Could you check a few things on this model? Use its own coordinates, in mm. Face numbers are marked on the shaded views. Round coordinates to 2 decimals unless told otherwise and drop trailing zeros. Loops run counter-clockwise (first coordinate to the right, second up) from the corner with the lowest first, then second, coordinate; pieces in that order, holes last. Notation, with made-up numbers: (-4, 21) -> (22, 21) arc R31 ccw to (22, 56) -> close; hole circle Ø10 at (76, -25). An arc over 180 degrees is marked (long way). Write each question's results on one line, items separated by ' | '. Start each with the question number.
1) Imagine slicing it at C-C, the plane y = 2.25. List the corners of the cut face in (x, z) for me.
2) We'd pull the mould along Y, two halves only. Please class the marked faces 1, 2 and 3: pulls with the +Y half, pulls with the -Y half, needs draft (parallel to the pull), parting line crosses it, or undercut.
3) If I drill on probe 1 along X at (y, z) = (-0.2, 3.17); probe 2 along X at (y, z) = (0.45, -1.91); probe 3 along Z at (x, y) = (4.5, -0.15), over which ranges is the centre line in solid material (lowest first)?
4) Imagine slicing it at D-D, the plane z = 0.63. Give the number of separate pieces and of enclosed holes in the cut face, plus the area to 3 significant figures.
5) Imagine slicing it at B-B, the plane x = 3.25. List the corners of the cut face in (y, z) for me.
6) Imagine slicing it at A-A, the plane z = -4.45. List the corners of the cut face in (x, y) for me, plus the area to 3 significant figures.
7) For P1, Ø1.5, axis at x = 0, z = -8, coming from the -Y side; P2, Ø1.8, axis at x = 7.5, z = 0.5, coming from the +Y side; P3, Ø2, axis at x = -6, y = 0.5, coming from the -Z side, each with a flat end and sliding along its axis, tell me the tip position at first contact or that it passes through.
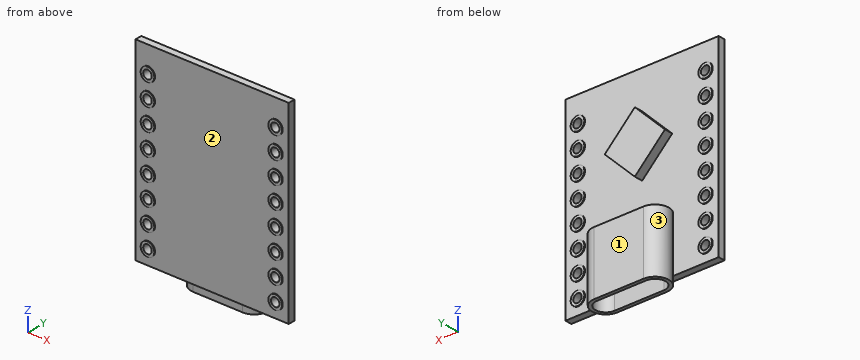
from build123d import *

# Parameters (mm, degrees)
SKETCH1_W                = 18
SKETCH1_H                = 22.5
BOSS_EXTRUDE1_DEPTH      = 0.4
CUT_EXTRUDE1_DEPTH       = 15.429223818
CUT_EXTRUDE1_DEPTH_BACK  = 15.429223818
SKETCH2_R                = 0.5
BOSS_EXTRUDE2_DEPTH      = 1.35
BOSS_EXTRUDE2_DEPTH_BACK = 6
CUT_EXTRUDE2_DEPTH       = 26.744562533
CUT_EXTRUDE2_DEPTH_BACK  = 7
BOSS_EXTRUDE3_DEPTH      = 1
BOSS_EXTRUDE4_DEPTH      = 0.1
BOSS_EXTRUDE4_DEPTH_BACK = 0.9
SKETCH6_R                = 0.8
SKETCH6_R_2              = 0.5


with BuildPart() as part:
    # Sketch1 → Boss-Extrude1 (new, symmetric)
    with BuildSketch(Plane(origin=(0, 0, 0), x_dir=(1, 0, 0), z_dir=(0, 1, 0))):
        Rectangle(SKETCH1_W, SKETCH1_H)
    extrude(amount=BOSS_EXTRUDE1_DEPTH, both=True)

    # Sketch2 → Cut-Extrude1 (cut, two sides: drawn at the far end of the back side and taken through both)
    with BuildSketch(Plane(origin=(0, 0.4, 0), x_dir=(1, 0, 0), z_dir=(0, 1, 0)).offset(-CUT_EXTRUDE1_DEPTH_BACK)):
        with Locations(Location((7.5, -8.25, 0), (0, 0, 270))):
            Circle(SKETCH2_R)
        with Locations(Location((-7.5, -8.25, 0), (0, 0, 270))):
            Circle(SKETCH2_R)
        with Locations(Location((-7.5, -5.71, 0), (0, 0, 270))):
            Circle(SKETCH2_R)
        with Locations(Location((7.5, -5.71, 0), (0, 0, 270))):
            Circle(SKETCH2_R)
        with Locations(Location((-7.5, -3.17, 0), (0, 0, 270))):
            Circle(SKETCH2_R)
        with Locations(Location((7.5, -3.17, 0), (0, 0, 270))):
            Circle(SKETCH2_R)
        with Locations(Location((-7.5, -0.63, 0), (0, 0, 270))):
            Circle(SKETCH2_R)
        with Locations(Location((7.5, -0.63, 0), (0, 0, 270))):
            Circle(SKETCH2_R)
        with Locations(Location((-7.5, 1.91, 0), (0, 0, 270))):
            Circle(SKETCH2_R)
        with Locations(Location((7.5, 1.91, 0), (0, 0, 270))):
            Circle(SKETCH2_R)
        with Locations(Location((-7.5, 4.45, 0), (0, 0, 270))):
            Circle(SKETCH2_R)
        with Locations(Location((7.5, 4.45, 0), (0, 0, 270))):
            Circle(SKETCH2_R)
        with Locations(Location((-7.5, 6.99, 0), (0, 0, 270))):
            Circle(SKETCH2_R)
        with Locations(Location((7.5, 6.99, 0), (0, 0, 270))):
            Circle(SKETCH2_R)
        with Locations(Location((-7.5, 9.53, 0), (0, 0, 270))):
            Circle(SKETCH2_R)
        with Locations(Location((7.5, 9.53, 0), (0, 0, 270))):
            Circle(SKETCH2_R)
    extrude(amount=CUT_EXTRUDE1_DEPTH + CUT_EXTRUDE1_DEPTH_BACK, mode=Mode.SUBTRACT)

    # Sketch3 → Boss-Extrude2 (add, two sides: drawn at the far end of the back side and taken through both)
    with BuildSketch(Plane(origin=(0, 0, -11.25), x_dir=(-1, 0, 0), z_dir=(0, 0, -1)).offset(-BOSS_EXTRUDE2_DEPTH_BACK)):
        with BuildLine():
            Line((-2.9, 3.6), (2.9, 3.6))
            ThreePointArc((2.9, 3.6), (4.5, 2), (2.9, 0.4))
            Line((2.9, 0.4), (-2.9, 0.4))
            ThreePointArc((-2.9, 0.4), (-4.5, 2), (-2.9, 3.6))
        make_face()
    extrude(amount=BOSS_EXTRUDE2_DEPTH + BOSS_EXTRUDE2_DEPTH_BACK)

    # Sketch4 → Cut-Extrude2 (cut, two sides: drawn at the far end of the back side and taken through both)
    with BuildSketch(Plane(origin=(0, 0, -12.6), x_dir=(-1, 0, 0), z_dir=(0, 0, -1)).offset(-CUT_EXTRUDE2_DEPTH_BACK)):
        with BuildLine():
            Line((-2.9, 0.8), (2.9, 0.8))
            ThreePointArc((2.9, 0.8), (4.1, 2), (2.9, 3.2))
            Line((2.9, 3.2), (-2.9, 3.2))
            ThreePointArc((-2.9, 3.2), (-4.1, 2), (-2.9, 0.8))
        make_face()
    extrude(amount=CUT_EXTRUDE2_DEPTH + CUT_EXTRUDE2_DEPTH_BACK, mode=Mode.SUBTRACT)

    # Sketch5 → Boss-Extrude3 (add)
    with BuildSketch(Plane(origin=(0, 0.4, 0), x_dir=(1, 0, 0), z_dir=(0, 1, 0))):
        Polygon((-3.542790315, -3.285533906), (-0.00725641, -6.821067812), (3.528277496, -3.285533906), (-0.00725641, 0.25), align=None)
    extrude(amount=BOSS_EXTRUDE3_DEPTH)

    # Sketch6 → Boss-Extrude4 (add, two sides: drawn at the far end of the back side and taken through both)
    # profile 1 of 16: a face of its own
    with BuildSketch(Plane(origin=(0, 0.4, 0), x_dir=(1, 0, 0), z_dir=(0, 1, 0)).offset(-BOSS_EXTRUDE4_DEPTH_BACK)):
        with Locations(Location((-7.5, -8.25, 0), (0, 0, 270))):
            Circle(SKETCH6_R)
        with Locations(Location((-7.5, -8.25, 0), (0, 0, 270))):
            Circle(SKETCH6_R_2, mode=Mode.SUBTRACT)
    # profile 2 of 16: a face of its own
    with BuildSketch(Plane(origin=(0, 0.4, 0), x_dir=(1, 0, 0), z_dir=(0, 1, 0)).offset(-BOSS_EXTRUDE4_DEPTH_BACK)):
        with Locations(Location((7.5, -8.25, 0), (0, 0, 270))):
            Circle(SKETCH6_R)
        with Locations(Location((7.5, -8.25, 0), (0, 0, 90))):
            Circle(SKETCH6_R_2, mode=Mode.SUBTRACT)
    # profile 3 of 16: a face of its own
    with BuildSketch(Plane(origin=(0, 0.4, 0), x_dir=(1, 0, 0), z_dir=(0, 1, 0)).offset(-BOSS_EXTRUDE4_DEPTH_BACK)):
        with Locations(Location((7.5, -5.71, 0), (0, 0, 270))):
            Circle(SKETCH6_R)
        with Locations(Location((7.5, -5.71, 0), (0, 0, 90))):
            Circle(SKETCH6_R_2, mode=Mode.SUBTRACT)
    # profile 4 of 16: a face of its own
    with BuildSketch(Plane(origin=(0, 0.4, 0), x_dir=(1, 0, 0), z_dir=(0, 1, 0)).offset(-BOSS_EXTRUDE4_DEPTH_BACK)):
        with Locations(Location((-7.5, -5.71, 0), (0, 0, 270))):
            Circle(SKETCH6_R)
        with Locations(Location((-7.5, -5.71, 0), (0, 0, 270))):
            Circle(SKETCH6_R_2, mode=Mode.SUBTRACT)
    # profile 5 of 16: a face of its own
    with BuildSketch(Plane(origin=(0, 0.4, 0), x_dir=(1, 0, 0), z_dir=(0, 1, 0)).offset(-BOSS_EXTRUDE4_DEPTH_BACK)):
        with Locations(Location((7.5, -3.17, 0), (0, 0, 270))):
            Circle(SKETCH6_R)
        with Locations(Location((7.5, -3.17, 0), (0, 0, 90))):
            Circle(SKETCH6_R_2, mode=Mode.SUBTRACT)
    # profile 6 of 16: a face of its own
    with BuildSketch(Plane(origin=(0, 0.4, 0), x_dir=(1, 0, 0), z_dir=(0, 1, 0)).offset(-BOSS_EXTRUDE4_DEPTH_BACK)):
        with Locations(Location((-7.5, -3.17, 0), (0, 0, 270))):
            Circle(SKETCH6_R)
        with Locations(Location((-7.5, -3.17, 0), (0, 0, 270))):
            Circle(SKETCH6_R_2, mode=Mode.SUBTRACT)
    # profile 7 of 16: a face of its own
    with BuildSketch(Plane(origin=(0, 0.4, 0), x_dir=(1, 0, 0), z_dir=(0, 1, 0)).offset(-BOSS_EXTRUDE4_DEPTH_BACK)):
        with Locations(Location((7.5, -0.63, 0), (0, 0, 270))):
            Circle(SKETCH6_R)
        with Locations(Location((7.5, -0.63, 0), (0, 0, 90))):
            Circle(SKETCH6_R_2, mode=Mode.SUBTRACT)
    # profile 8 of 16: a face of its own
    with BuildSketch(Plane(origin=(0, 0.4, 0), x_dir=(1, 0, 0), z_dir=(0, 1, 0)).offset(-BOSS_EXTRUDE4_DEPTH_BACK)):
        with Locations(Location((-7.5, -0.63, 0), (0, 0, 270))):
            Circle(SKETCH6_R)
        with Locations(Location((-7.5, -0.63, 0), (0, 0, 270))):
            Circle(SKETCH6_R_2, mode=Mode.SUBTRACT)
    # profile 9 of 16: a face of its own
    with BuildSketch(Plane(origin=(0, 0.4, 0), x_dir=(1, 0, 0), z_dir=(0, 1, 0)).offset(-BOSS_EXTRUDE4_DEPTH_BACK)):
        with Locations(Location((7.5, 1.91, 0), (0, 0, 270))):
            Circle(SKETCH6_R)
        with Locations(Location((7.5, 1.91, 0), (0, 0, 90))):
            Circle(SKETCH6_R_2, mode=Mode.SUBTRACT)
    # profile 10 of 16: a face of its own
    with BuildSketch(Plane(origin=(0, 0.4, 0), x_dir=(1, 0, 0), z_dir=(0, 1, 0)).offset(-BOSS_EXTRUDE4_DEPTH_BACK)):
        with Locations(Location((-7.5, 1.91, 0), (0, 0, 270))):
            Circle(SKETCH6_R)
        with Locations(Location((-7.5, 1.91, 0), (0, 0, 270))):
            Circle(SKETCH6_R_2, mode=Mode.SUBTRACT)
    # profile 11 of 16: a face of its own
    with BuildSketch(Plane(origin=(0, 0.4, 0), x_dir=(1, 0, 0), z_dir=(0, 1, 0)).offset(-BOSS_EXTRUDE4_DEPTH_BACK)):
        with Locations(Location((7.5, 4.45, 0), (0, 0, 270))):
            Circle(SKETCH6_R)
        with Locations(Location((7.5, 4.45, 0), (0, 0, 90))):
            Circle(SKETCH6_R_2, mode=Mode.SUBTRACT)
    # profile 12 of 16: a face of its own
    with BuildSketch(Plane(origin=(0, 0.4, 0), x_dir=(1, 0, 0), z_dir=(0, 1, 0)).offset(-BOSS_EXTRUDE4_DEPTH_BACK)):
        with Locations(Location((-7.5, 4.45, 0), (0, 0, 270))):
            Circle(SKETCH6_R)
        with Locations(Location((-7.5, 4.45, 0), (0, 0, 270))):
            Circle(SKETCH6_R_2, mode=Mode.SUBTRACT)
    # profile 13 of 16: a face of its own
    with BuildSketch(Plane(origin=(0, 0.4, 0), x_dir=(1, 0, 0), z_dir=(0, 1, 0)).offset(-BOSS_EXTRUDE4_DEPTH_BACK)):
        with Locations(Location((7.5, 6.99, 0), (0, 0, 270))):
            Circle(SKETCH6_R)
        with Locations(Location((7.5, 6.99, 0), (0, 0, 90))):
            Circle(SKETCH6_R_2, mode=Mode.SUBTRACT)
    # profile 14 of 16: a face of its own
    with BuildSketch(Plane(origin=(0, 0.4, 0), x_dir=(1, 0, 0), z_dir=(0, 1, 0)).offset(-BOSS_EXTRUDE4_DEPTH_BACK)):
        with Locations(Location((-7.5, 6.99, 0), (0, 0, 270))):
            Circle(SKETCH6_R)
        with Locations(Location((-7.5, 6.99, 0), (0, 0, 270))):
            Circle(SKETCH6_R_2, mode=Mode.SUBTRACT)
    # profile 15 of 16: a face of its own
    with BuildSketch(Plane(origin=(0, 0.4, 0), x_dir=(1, 0, 0), z_dir=(0, 1, 0)).offset(-BOSS_EXTRUDE4_DEPTH_BACK)):
        with Locations(Location((7.5, 9.53, 0), (0, 0, 270))):
            Circle(SKETCH6_R)
        with Locations(Location((7.5, 9.53, 0), (0, 0, 90))):
            Circle(SKETCH6_R_2, mode=Mode.SUBTRACT)
    # profile 16 of 16: a face of its own
    with BuildSketch(Plane(origin=(0, 0.4, 0), x_dir=(1, 0, 0), z_dir=(0, 1, 0)).offset(-BOSS_EXTRUDE4_DEPTH_BACK)):
        with Locations(Location((-7.5, 9.53, 0), (0, 0, 270))):
            Circle(SKETCH6_R)
        with Locations(Location((-7.5, 9.53, 0), (0, 0, 270))):
            Circle(SKETCH6_R_2, mode=Mode.SUBTRACT)
    extrude(amount=BOSS_EXTRUDE4_DEPTH + BOSS_EXTRUDE4_DEPTH_BACK)


solid = part.part
Checked values:
1) outline: (-4.48, -12.6) -> (-4.07, -12.6) -> (-4.07, -5.6) -> (4.07, -5.6) -> (4.07, -12.6) -> (4.48, -12.6) -> (4.48, -5.25) -> (-4.48, -5.25) -> close
2) face 1: pulls with the +Y half | face 2: pulls with the -Y half | face 3: undercut
3) probe 1: -9 to -8, -7 to 7, 8 to 9 | probe 2: -8.3 to -8, -7 to -6.7, 6.7 to 7, 8 to 8.3 | probe 3: -11.25 to 11.25
4) separate pieces: 3 | enclosed holes: 0 | area: 14.8 mm^2
5) outline: (-0.4, -11.25) -> (0.4, -11.25) -> (0.4, 3.01) -> (1.4, 3.01) -> (1.4, 3.56) -> (0.4, 3.56) -> (0.4, 11.25) -> (-0.4, 11.25) -> close; (0.44, -12.6) -> (0.85, -12.6) -> (0.85, -5.6) -> (3.15, -5.6) -> (3.15, -12.6) -> (3.56, -12.6) -> (3.56, -5.25) -> (0.44, -5.25) -> close
6) outline: (-9, -0.4) -> (-8.3, -0.4) -> (-8.3, -0.5) -> (-8, -0.5) -> (-8, 0.5) -> (-8.3, 0.5) -> (-8.3, 0.4) -> (-9, 0.4) -> close; (-7, -0.5) -> (-6.7, -0.5) -> (-6.7, -0.4) -> (6.7, -0.4) -> (6.7, -0.5) -> (7, -0.5) -> (7, 0.5) -> (6.7, 0.5) -> (6.7, 0.4) -> (-6.7, 0.4) -> (-6.7, 0.5) -> (-7, 0.5) -> close; (8, -0.5) -> (8.3, -0.5) -> (8.3, -0.4) -> (9, -0.4) -> (9, 0.4) -> (8.3, 0.4) -> (8.3, 0.5) -> (8, 0.5) -> close | area: 13.0 mm^2
7) P1: y = -0.4 | P2: y = 0.5 | P3: z = -11.25
